```python
from build123d import *

# Parameters (mm, degrees)
F0_R     = 12.7
F0_R_2   = 7.9375
F1_DEPTH = 19.05
F2_R     = 9.525
F2_R_2   = 7.9375
F3_DEPTH = 15.875
F4_R     = 15.875
F4_R_2   = 12.7
F5_DEPTH = 3.175
F6_R     = 15.875
F6_R_2   = 12.7
F7_DEPTH = 3.175


with BuildPart() as f1:
    # F0 (on Top) → F1 (new body)
    with BuildSketch(Plane.XY):
        Circle(F0_R)
        Circle(F0_R_2, mode=Mode.SUBTRACT)
    extrude(amount=F1_DEPTH)

    # F2 (on face) → F3 (cut)
    with BuildSketch(Plane.XY.offset(19.05)):
        Circle(F2_R)
        Circle(F2_R_2, mode=Mode.SUBTRACT)
    extrude(amount=-F3_DEPTH, mode=Mode.SUBTRACT)

    # F4 (on face) → F5 (join)
    with BuildSketch(Plane.XY.offset(3.175)):
        Circle(F4_R)
        Circle(F4_R_2, mode=Mode.SUBTRACT)
    extrude(amount=-F5_DEPTH)

    # F6 (on face) → F7 (join)
    with BuildSketch(Plane.XY.offset(19.05)):
        Circle(F6_R)
        Circle(F6_R_2, mode=Mode.SUBTRACT)
    extrude(amount=-F7_DEPTH)


solid = f1.part
```
Source: CAD feature listing. Evaluate the final solid. Frame: model axes, mm. A direction names the side the tool comes from. Coordinates: 2 decimals unless noted, no trailing zeros. Loops run counter-clockwise (first coordinate to the right, second up) from the corner with the lowest first, then second, coordinate; pieces in that order, holes last. Notation, with made-up numbers: M -4.75,8 L 2.25,8 A27 cw 2.25,31 Z; hole C 81,19 d7. An arc over 180 degrees is marked long. Use a Markdown table: item, result. Add a question column.
Q1. Section query D-D, the plane y = -10. Return loops of the section in (x, z) (3 decimals), and give its area (3 significant figures).
Q2. Access query for faces 1 (the cylindrical face through (-2.75, -12.4, 9.44)), 2 (the flat face through (-3.8, 7.3, 0)), 3 (the cylindrical face through (-7.559, -5.796, 11.224)). Directions: +Z, -Z, +X, -X, +Y, -Y. A direction counts if a zero-diameter tool reaches every point of the face in a straight line with its end or side. Return the directions, or none.
Q3. Material intervals for L1, parallel to Y at x = 0, z = 15.5 (3 decimals); L2, parallel to Z at x = 3, y = -13 (3 decimals); L3, parallel to X at y = 4, z = 13.5, sorted ascending.
Q4. Section query C-C, the plane z = 3.75. Return loops of the section in (x, y) (3 decimals), and give its area (3 significant figures).
Q5. Draft query along Y for faces 4 (the cylindrical face through (-3.441, -15.497, 1.61)), 5 (the flat face through (-2, 8, 3.175)), 6 (the flat face through (-7, 11, 15.875)). Return one class per face: pulls with the +Y half, pulls with the -Y half, needs draft (parallel to the pull), parting line crosses it, or undercut.
Q6. First-contact query: pin 1 (12.5 mm diameter, centred on x = 0, y = 0, fed in from -Z); pin 2 (8 mm diameter, centred on x = 5, y = -6, fed in from +Z); pin 3 (10 mm diameter, centred on y = -10, z = 3.5, fed in from -X); pin 4 (2 mm diameter, centred on y = -6, z = 16, fed in from +X). Flat tips, straight axial feed; report the tip coordinate or a pass-through.
Result:
| question | item | result |
|---|---|---|
| 1 | outline | M -12.329,0 L 12.329,0 L 12.329,3.175 L 7.829,3.175 L 7.829,15.875 L 12.329,15.875 L 12.329,19.05 L -12.329,19.05 L -12.329,15.875 L -7.829,15.875 L -7.829,3.175 L -12.329,3.175 Z |
| 1 | area | 355 mm2 |
| 2 | face 1 | none |
| 2 | face 2 | -Z, +X, -X, +Y, -Y |
| 2 | face 3 | +Z |
| 3 | L1 | y = -12.7 to -9.525, 9.525 to 12.7 |
| 3 | L2 | z = 0 to 3.175, 15.875 to 19.05 |
| 3 | L3 | x = -12.05 to -8.64, 8.64 to 12.05 |
| 4 | outline | C 0,0 d25.4; hole C 0,0 d19.05 |
| 4 | area | 222 mm2 |
| 5 | face 4 | parting line crosses it |
| 5 | face 5 | undercut |
| 5 | face 6 | needs draft |
| 6 | pin 1 | passes through |
| 6 | pin 2 | stops at z = 19.05 |
| 6 | pin 3 | stops at x = -15.06 |
| 6 | pin 4 | stops at x = 15.07 |
